```python
from build123d import *

# Parameters (mm, degrees)
SKETCH1_R               = 2
SKETCH1_R_2             = 7.5
SKETCH1_R_3             = 2.5
BOSS_EXTRUDE1_DEPTH     = 3
CUT_EXTRUDE1_DEPTH      = 430.43916915
CUT_EXTRUDE1_DEPTH_BACK = 430.43916915
CUT_EXTRUDE2_DEPTH      = 430.43916915
CUT_EXTRUDE2_DEPTH_BACK = 430.43916915
SKETCH5_R               = 2.5
CUT_EXTRUDE3_DEPTH      = 430.43916915
CUT_EXTRUDE3_DEPTH_BACK = 430.43916915
SKETCH6_R               = 1.500000001
SKETCH6_R_2             = 1.5
SKETCH6_R_3             = 1.499999999
SKETCH7_R               = 1.5
CUT_EXTRUDE4_DEPTH      = 3
CUT_EXTRUDE5_DEPTH      = 430.43916915


with BuildPart() as part:
    # Sketch1 → Boss-Extrude1 (new body)
    with BuildSketch(Plane.XY):
        with BuildLine():
            Line((0, 35), (0, -35))
            Line((0, -35), (393, -35))
            ThreePointArc((393, -35), (428, 0), (393, 35))
            Line((393, 35), (0, 35))
        make_face()
        with Locations((5, 29)):
            Circle(SKETCH1_R, mode=Mode.SUBTRACT)
        with Locations(Location((5, -29, 0), (0, 0, 180))):
            Circle(SKETCH1_R, mode=Mode.SUBTRACT)
        with Locations((393, 0)):
            Circle(SKETCH1_R_2, mode=Mode.SUBTRACT)
        with Locations((103, 0)):
            Circle(SKETCH1_R_3, mode=Mode.SUBTRACT)
        with Locations((31, 29)):
            Circle(SKETCH1_R, mode=Mode.SUBTRACT)
        with Locations((31, -29)):
            Circle(SKETCH1_R, mode=Mode.SUBTRACT)
        with Locations((5, 0)):
            Circle(SKETCH1_R, mode=Mode.SUBTRACT)
    extrude(amount=BOSS_EXTRUDE1_DEPTH)

    # Sketch4 → Cut-Extrude1 (cut, two sides: drawn at the far end of the back side and taken through both)
    with BuildSketch(Plane.XY.offset(3).offset(-CUT_EXTRUDE1_DEPTH_BACK)):
        with BuildLine():
            Line((55.5, 27), (55.5, 12))
            ThreePointArc((55.5, 12), (53, 9.5), (50.5, 12))
            Line((50.5, 12), (50.5, 27))
            ThreePointArc((50.5, 27), (53, 29.5), (55.5, 27))
        make_face()
        with BuildLine():
            Line((155.5, 22), (155.5, 7))
            ThreePointArc((155.5, 7), (153, 4.5), (150.5, 7))
            Line((150.5, 7), (150.5, 22))
            ThreePointArc((150.5, 22), (153, 24.5), (155.5, 22))
        make_face()
        with BuildLine():
            Line((155.5, -22), (155.5, -7))
            ThreePointArc((155.5, -7), (153, -4.5), (150.5, -7))
            Line((150.5, -7), (150.5, -22))
            ThreePointArc((150.5, -22), (153, -24.5), (155.5, -22))
        make_face()
        with BuildLine():
            Line((55.5, -27), (55.5, -12))
            ThreePointArc((55.5, -12), (53, -9.5), (50.5, -12))
            Line((50.5, -12), (50.5, -27))
            ThreePointArc((50.5, -27), (53, -29.5), (55.5, -27))
        make_face()
    extrude(amount=CUT_EXTRUDE1_DEPTH + CUT_EXTRUDE1_DEPTH_BACK, mode=Mode.SUBTRACT)

    # Sketch5 → Cut-Extrude2 (cut, two sides: drawn at the far end of the back side and taken through both)
    with BuildSketch(Plane.XY.offset(3).offset(-CUT_EXTRUDE2_DEPTH_BACK)):
        with Locations((335.5, 0)):
            Circle(SKETCH5_R)
    extrude(amount=CUT_EXTRUDE2_DEPTH + CUT_EXTRUDE2_DEPTH_BACK, mode=Mode.SUBTRACT)

    # Sketch6 → Cut-Extrude3 (cut, two sides: drawn at the far end of the back side and taken through both)
    with BuildSketch(Plane.XY.offset(3).offset(-CUT_EXTRUDE3_DEPTH_BACK)):
        with Locations((420.999999999, 1e-09)):
            Circle(SKETCH6_R)
        with Locations((393, -27.999999998)):
            Circle(SKETCH6_R_2)
        with Locations((393, 28)):
            Circle(SKETCH6_R_2)
        with Locations((365.000000001, 1e-09)):
            Circle(SKETCH6_R_3)
    extrude(amount=CUT_EXTRUDE3_DEPTH + CUT_EXTRUDE3_DEPTH_BACK, mode=Mode.SUBTRACT)

    # Sketch7 → Cut-Extrude4 (cut)
    with BuildSketch(Plane.XY.offset(3)):
        with Locations((73, 29)):
            Circle(SKETCH7_R)
        with Locations((133, 29)):
            Circle(SKETCH7_R)
        with Locations((193, 29)):
            Circle(SKETCH7_R)
        with Locations((253, 29)):
            Circle(SKETCH7_R)
        with Locations((313, 29)):
            Circle(SKETCH7_R)
        with Locations((358, 29)):
            Circle(SKETCH7_R)
    extrude(amount=-CUT_EXTRUDE4_DEPTH, mode=Mode.SUBTRACT)

    # Sketch8 → Cut-Extrude5 (cut, through all)
    with BuildSketch(Plane.XY.offset(3)):
        Polygon((223.795, 0), (218.021497308, 10), (206.474491924, 10), (200.700989232, 0), (206.474491924, -10), (218.021497308, -10), align=None)
        Polygon((191.795, 0), (186.021497308, 10), (174.474491924, 10), (168.700989232, 0), (174.474491924, -10), (186.021497308, -10), align=None)
        Polygon((255.795, 0), (250.021497308, 10), (238.474491924, 10), (232.700989232, 0), (238.474491924, -10), (250.021497308, -10), align=None)
        Polygon((287.795, 0), (282.021497308, 10), (270.474491924, 10), (264.700989232, 0), (270.474491924, -10), (282.021497308, -10), align=None)
        Polygon((233.865777575, 16), (231.056886095, 20.865142755), (225.439103137, 20.865142755), (222.630211658, 16), (225.439103137, 11.134857245), (231.056886095, 11.134857245), align=None)
        Polygon((201.865777575, 16), (199.056886095, 20.865142755), (193.439103137, 20.865142755), (190.630211658, 16), (193.439103137, 11.134857245), (199.056886095, 11.134857245), align=None)
        Polygon((265.865777575, 16), (263.056886095, 20.865142755), (257.439103137, 20.865142755), (254.630211658, 16), (257.439103137, 11.134857245), (263.056886095, 11.134857245), align=None)
        Polygon((319.795, 0), (314.021497308, 10), (302.474491924, 10), (296.700989232, 0), (302.474491924, -10), (314.021497308, -10), align=None)
        Polygon((297.865777575, 16), (295.056886095, 20.865142755), (289.439103137, 20.865142755), (286.630211658, 16), (289.439103137, 11.134857245), (295.056886095, 11.134857245), align=None)
        Polygon((295.056886095, -11.134857245), (297.865777575, -16), (295.056886095, -20.865142755), (289.439103137, -20.865142755), (286.630211658, -16), (289.439103137, -11.134857245), align=None)
        Polygon((263.056886095, -11.134857245), (265.865777575, -16), (263.056886095, -20.865142755), (257.439103137, -20.865142755), (254.630211658, -16), (257.439103137, -11.134857245), align=None)
        Polygon((231.056886095, -11.134857245), (233.865777575, -16), (231.056886095, -20.865142755), (225.439103137, -20.865142755), (222.630211658, -16), (225.439103137, -11.134857245), align=None)
        Polygon((199.056886095, -11.134857245), (201.865777575, -16), (199.056886095, -20.865142755), (193.439103137, -20.865142755), (190.630211658, -16), (193.439103137, -11.134857245), align=None)
    extrude(amount=-CUT_EXTRUDE5_DEPTH, mode=Mode.SUBTRACT)


solid = part.part
```
CAD build for the part. Positions are in the model's coordinates, mm. Coordinates: 2 decimals unless noted, no trailing zeros. Write each loop counter-clockwise with the first axis right and the second up, starting at its lowest first coordinate (ties: lowest second). Pieces come first, ordered by that corner, then holes.
(1) Two-plate mould, pull along Y, no slides. Class faces 1 (the face through (427.99, -0.77, 1.48)), 2 (the face through (211, 16, 0)), 3 (the face through (399.93, -2.87, 1.48)): +Y half, -Y half, draft (parallel to the pull), parting line (faces both ways), or undercut.
(2) Cut at B-B, the plane z = 1.1. Count the separate pieces of the cut face and the enclosed holes in it, and give its area (3 significant figures).
(3) Cut at A-A, the plane x = 275.5. List the corners of the cut face in (y, z).
(4) Drill centre lines: probe 1 along Y at (x, z) = (5, 0.95); probe 2 along Y at (x, z) = (133, 1.25); probe 3 along Y at (x, z) = (103, 0.8). Where is each one in solid material? Low to high.
Geometry says:
1. face 1: parting line
1. face 2: draft
1. face 3: undercut
2. separate pieces: 1
2. enclosed holes: 35
2. area: 26,300 mm2
3. outline: (-35, 0) - (-10, 0) - (-10, 3) - (-35, 3) - close; (10, 0) - (35, 0) - (35, 3) - (10, 3) - close
4. probe 1: y = -35 to -31, -27 to -2, 2 to 27, 31 to 35
4. probe 2: y = -35 to 27.5, 30.5 to 35
4. probe 3: y = -35 to -2.5, 2.5 to 35
